Work out the finished part from the listing and answer in its coordinate system (mm). A direction names the side the tool comes from. Give positions to 0.01 mm unless a question says otherwise; leave off trailing zeros. Loops run counter-clockwise (first coordinate to the right, second up) from the corner with the lowest first, then second, coordinate; pieces in that order, holes last. Notation, with made-up numbers: (61, -24) - (65, -24) arc R6 cw to (65, -14) - close; hole circle Ø6 at (39.5, 43.25). An arc over 180 degrees is marked (long way). One line per question, with ' | ' between items.
from build123d import *

# Parameters (mm, degrees)
F2_R     = 6.8
F3_DEPTH = 5.7
F4_R     = 3
F5_DEPTH = 0.5


with BuildPart() as f1:
    # F0 (on Front) → F1 (revolve)
    with BuildSketch(Plane.XZ):
        with BuildLine():
            Line((-10.1, 0), (0, 0))
            Line((0, 0), (0, 7.1))
            ThreePointArc((0, 7.1), (-3.641772, 6.823414), (-7.2, 6))
            Line((-7.2, 6), (-7.2, 2.5))
            Line((-7.2, 2.5), (-10.1, 2.5))
            Line((-10.1, 2.5), (-10.1, 0))
        make_face()
    revolve(axis=Axis((0, 0, 3.55), (0, 0, -1)))

    # F2 (on face) → F3 (cut)
    with BuildSketch(Plane(origin=(0, 0, 0), x_dir=(1, 0, 0), z_dir=(0, 0, -1))):
        Circle(F2_R)
    extrude(amount=-F3_DEPTH, mode=Mode.SUBTRACT)

    # F4 (on face) → F5 (join)
    with BuildSketch(Plane(origin=(0, 0, 5.7), x_dir=(1, 0, 0), z_dir=(0, 0, -1))):
        Circle(F4_R)
    extrude(amount=F5_DEPTH)


solid = f1.part
1. Determine the mould class of faces 1 (the cylindrical face through (-6.87, 2.16, 4.23)), 2 (the flat face through (4, -7, 2.5)), 3 (the cylindrical face through (-1.47, 6.64, 2.81)) for opening direction Y: +Y half, -Y half, draft (parallel to the pull), parting line (faces both ways), or undercut.
Evaluation:
face 1: parting line | face 2: draft | face 3: undercut
2. Find section B-B on z = 4.75. Write down the section's boundary in (x, y), then the cut area to 3 significant figures.
Evaluation:
outline: circle Ø14.4 at (0, 0); hole circle Ø13.6 at (0, 0) | area: 17.6 mm2
3. Flat-ended cylindrical pins translate along their axes: pin 1 (1 mm diameter, centred on x = 3.5, y = 5, fed in from -Z); pin 2 (11 mm diameter, centred on x = 0.5, y = -0.5, fed in from -Z); pin 3 (1.5 mm diameter, centred on x = 4.5, y = 4, fed in from +Z). Find the tip coordinate at first contact, or state that the pin passes through.
Evaluation:
pin 1: z = 5.7 | pin 2: z = 5.2 | pin 3: z = 6.52
4. Find section A-A on z = 2.25. Write down the section's boundary in (x, y), then the cut area to 3 significant figures.
Evaluation:
outline: circle Ø20.2 at (0, 0); hole circle Ø13.6 at (0, 0) | area: 175 mm2
5. Consider L1, parallel to Y at x = 0, z = 4.25; L2, parallel to Z at x = 8.5, y = -4.25; L3, parallel to Y at x = -3.75, z = 3. Determine where each line is inside the solid, lowest interval first.
Evaluation:
L1: -7.2 to -6.8, 6.8 to 7.2 | L2: 0 to 2.5 | L3: -6.15 to -5.67, 5.67 to 6.15
6. Which of the six approach directions +Z, -Z, +X, -X, +Y, -Y give full straight-line access (tool end or side, diameter ignored) to faces 4 (the cylindrical face through (-9.634, 3.034, 1.232)), 5 (the flat face through (3, 1, 5.7))?
Evaluation:
face 4: +Z, -Z | face 5: -Z
